Drawing for the job (mm, zero at the part's lowest x, y, z). A direction names the side the tool comes from. Coordinates: 2 decimals unless noted, no trailing zeros. Write each loop counter-clockwise with the first axis right and the second up, starting at its lowest first coordinate (ties: lowest second). Pieces come first, ordered by that corner, then holes. Notation, with made-up numbers: (16.25, 52.5) - (52.25, 52.5) arc R26 ccw to (52.25, 86.5) - close; hole circle Ø3 at (26, 22). An arc over 180 degrees is marked (long way). Write each question's results on one line, items separated by ' | '.
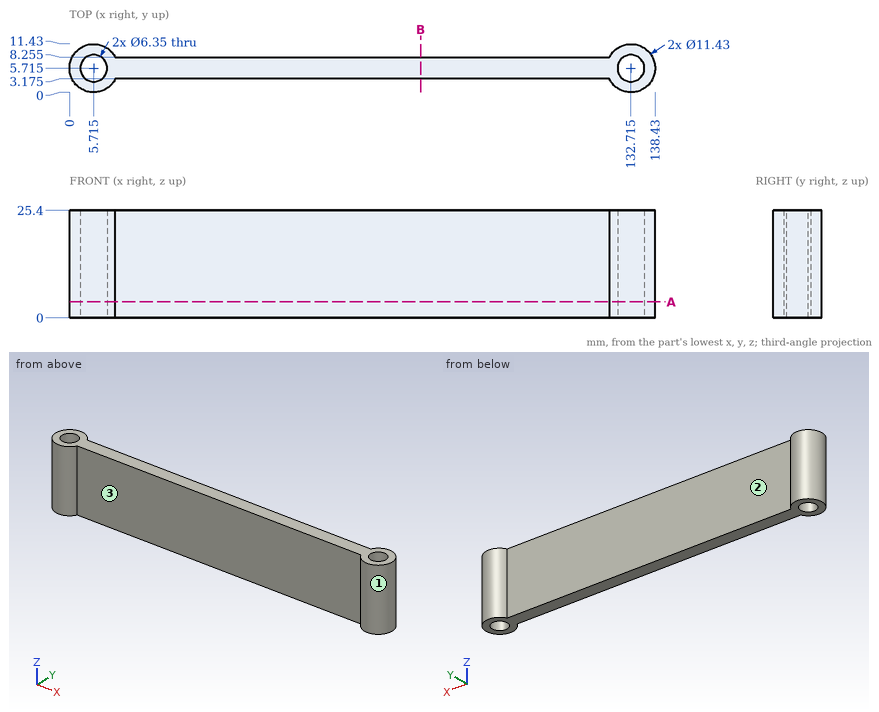
(1) Wall check: line 1 (X direction, y = 5.75, z = 21.5); line 2 (X direction, y = 6, z = 7.25); line 3 (X direction, y = 8.5, z = 22.25). Give the ranges that are in metal, low to high. Write a range as from..to.
Return value:
line 1: x = 0..2.54, 8.89..129.54, 135.89..138.43 | line 2: x = 0.01..2.55, 8.88..129.55, 135.88..138.42 | line 3: x = 0.72..4.19, 7.24..10.71, 127.72..131.19, 134.24..137.71
(2) Saw through at A-A on z = 3.75. Write the cut outline in (x, y) (3 decimals), then the cut area to 3 significant figures.
Return value:
outline: (10.835, 3.175) - (127.595, 3.175) arc R5.715 ccw (long way) to (127.595, 8.255) - (10.835, 8.255) arc R5.715 ccw (long way) to start; hole circle Ø6.35 at (5.715, 5.715); hole circle Ø6.35 at (132.715, 5.715) | area: 731 mm^2
(3) Flat gauge pins, fed straight in: P1, Ø2, axis at y = 9.5, z = 20.5, coming from the -X side; P2, Ø1.5, axis at x = 107, z = 14, coming from the -Y side (3 decimals); P3, Ø7.5, axis at x = 85.5, z = 9.5, coming from the +Y side (3 decimals). Where does each tip first touch, or does it go through?
Return value:
P1: stops at x = 0.72 | P2: stops at y = 3.175 | P3: stops at y = 8.255
(4) Saw through at B-B on x = 83. Write the cut outline in (y, z) (3 decimals), then the cut area to 3 significant figures.
Return value:
outline: (3.175, 0) - (8.255, 0) - (8.255, 25.4) - (3.175, 25.4) - close | area: 129 mm^2
(5) 3-axis set-ups, long thin cutter, end or side, ignore diameter. For the marked faces 1, 2 and 3: which of +Z, -Z, +X, -X, +Y, -Y reach the whole face in a straight line?
Return value:
face 1: +Z, -Z | face 2: +Z, -Z, +Y | face 3: +Z, -Z, -Y
